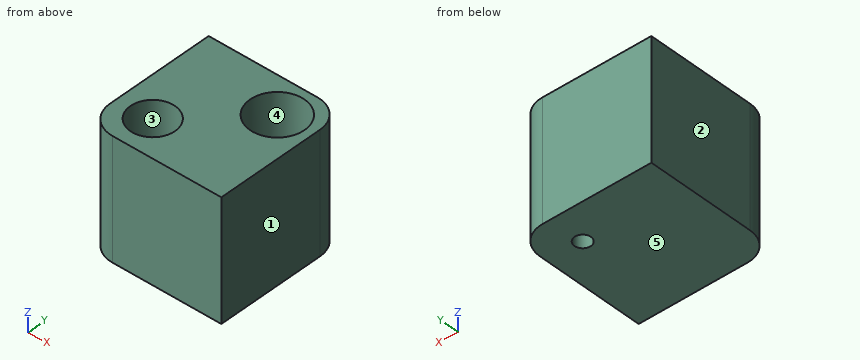
Autodesk Inventor part; units mm, degrees
ref_plane "YZ Plane" through (0, 0, 0) normal (1, 0, 0) x (0, 1, 0)
ref_plane "XZ Plane" through (0, 0, 0) normal (0, 1, 0) x (-1, 0, 0)
ref_plane "XY Plane" through (0, 0, 0) normal (0, 0, 1) x (1, 0, 0)
sketch "Sketch1" plane through (0, 0, 0) normal (0, 0, 1) x (1, 0, 0)
  line L0 (5, 0) -> (25, 0)
  line L1 (25, 0) -> (25, 20)
  line L2 (20, 25) -> (0, 25)
  line L3 (0, 25) -> (0, 5)
  arc A0 (25, 20) -> (20, 25) centre (20, 20) ccw
  arc A1 (0, 5) -> (5, 0) centre (5, 5) ccw
  point P0 (0, 0)
  point P1 (25, 25)
  dimension "d0" = 25
  dimension "d1" = 25
  dimension "d2" = 5
  dimension "d29" = 5
extrude "Extrusion1" add sketch "Sketch1" along normal blind 22
sketch "Sketch2" plane through (0, 0, 22) normal (0, 0, 1) x (1, 0, 0)
  line L0 (20, 25) -> (0, 25)
  line L1 (25, 0) -> (25, 20)
  point P0 (0, 0)
  point P1 (18.5, 18.5)
  dimension "d12" = 6.5
  dimension "d13" = 6.5
hole "Hole1" at (18.5, 18.5, 22) direction (0, 0, -1) diameter 10 depth 16
sketch "Sketch3" plane through (18.5, 18.5, 6) normal (0, 0, 1) x (1, 0, 0)
  line L0 (6.5, -18.5) -> (6.5, 1.5)
  line L1 (1.5, 6.5) -> (-18.5, 6.5)
  point P0 (-18.5, -18.5)
  point P1 (0, 0)
  dimension "d21" = 6.5
  dimension "d22" = 6.5
hole "Hole2" at (18.5, 18.5, 6) direction (0, 0, -1) diameter 3 depth 15
chamfer "Chamfer2" distance 2 angle 45 1 edges at (18.5, 20, 6)
sketch "Sketch4" plane through (0, 0, 22) normal (0, 0, 1) x (1, 0, 0)
  line L0 (5, 0) -> (25, 0)
  line L1 (0, 25) -> (0, 5)
  point P0 (0, 0)
  point P1 (6.5, 6.5)
  dimension "d37" = 6.5
  dimension "d38" = 6.5
hole "Hole3" at (6.5, 6.5, 22) direction (0, 0, -1) diameter 8.2 depth 16
properties part number "spacer dubbele hoogte behuizing"
Check sheet for the modelled part. Datum: model origin and axes. Units: mm. Face numbers are marked on the shaded views. A direction names the side the tool comes from. Coordinates: 2 decimals unless noted, no trailing zeros. Order: outer loops, then holes, each group sorted by start corner. A loop starts at its lowest first (then second) coordinate and runs counter-clockwise, first axis right, second up. Notation, with made-up numbers: (31.25, 7.5) -> (59.25, 7.5) arc R19 ccw to (59.25, 24.5) -> close; hole circle Ø10 at (-31, 84.5). An arc over 180 degrees is marked (long way). Write item = value, one per line. Start each with the question number.
1) Cross-section at D-D (y = 6.5). Enter the section's corners in (x, z).
2) Access from +Z, -Z, +X, -X, +Y, -Y to the whole of each face (thin tool, end or side, straight path). Record for the marked faces 4 and 5.
3) Go/stop test with a flat-tipped pin: P1, Ø6.5, axis at x = 7.5, y = 5, coming from the +Z side. Record where the tip stops, or that it passes through.
4) Mould release check, pull along X, two halves, no side actions. Record for the marked faces 1, 2 and 3: +X half, -X half, draft (parallel to the pull), parting line (faces both ways), or undercut.
5) Cross-section at A-A (z = 14.5). Enter the section's corners in (x, y), then the cut area to 3 significant figures.
6) Material ranges on L1, parallel to Y at x = 18.5, z = 18.5; L2, parallel to Y at x = 18.5, z = 1.95, recorded low to high.
7) Cross-section at C-C (z = 5.5). Enter the section's corners in (x, y), then the cut area to 3 significant figures.
8) Cross-section at B-B (x = 18.5). Enter the section's corners in (y, z), then the cut area to 3 significant figures.
Ans:
q1.outline = (0, 0) -> (25, 0) -> (25, 22) -> (10.6, 22) -> (10.6, 6) -> (2.4, 6) -> (2.4, 22) -> (0, 22) -> close
q2.face_4 = +Z
q2.face_5 = -Z, +X, -X, +Y, -Y
q3.P1 = 22
q4.face_1 = +X half
q4.face_2 = -X half
q4.face_3 = undercut
q5.outline = (0, 5) arc R5 ccw to (5, 0) -> (25, 0) -> (25, 20) arc R5 ccw to (20, 25) -> (0, 25) -> close; hole circle Ø8.2 at (6.5, 6.5); hole circle Ø10 at (18.5, 18.5)
q5.area = 483 mm²
q6.L1 = 0 to 13.5, 23.5 to 25
q6.L2 = 0 to 17, 20 to 25
q7.outline = (0, 5) arc R5 ccw to (5, 0) -> (25, 0) -> (25, 20) arc R5 ccw to (20, 25) -> (0, 25) -> close; hole circle Ø6 at (18.5, 18.5)
q7.area = 586 mm²
q8.outline = (0, 0) -> (17, 0) -> (17, 4) -> (15, 6) -> (13.5, 6) -> (13.5, 22) -> (0, 22) -> close; (20, 0) -> (25, 0) -> (25, 22) -> (23.5, 22) -> (23.5, 6) -> (22, 6) -> (20, 4) -> close
q8.area = 368 mm²
